For this review, take the finished solid that the model builds, in its own axes (mm). Face numbers are marked on the shaded views. A direction names the side the tool comes from. Round coordinates to 2 decimals unless told otherwise and drop trailing zeros. Loops run counter-clockwise (first coordinate to the right, second up) from the corner with the lowest first, then second, coordinate; pieces in that order, holes last. Notation, with made-up numbers: (-38.5, 53.25) -> (-26.5, 53.25) arc R28 cw to (-26.5, 91.25) -> close; hole circle Ø3 at (16.25, -18). An arc over 180 degrees is marked (long way). One line per question, with ' | ' between items. Start each with the question number.
1. Consider section A-A (x = -139.7). Write out the cut boundary in (y, z) (3 decimals).
2. Consider section B-B (z = -25.4). Write out the cut boundary in (x, y) (3 decimals), and give its area (3 significant figures).
3. Consider section C-C (x = -158.75). Write out the cut boundary in (y, z) (3 decimals).
4. For the marked faces 1 and 2, list the 3-axis set-ups (+Z, -Z, +X, -X, +Y, -Y) from which the entire face can be reached by the end or side of a thin tool; tool diameter is ignored.
5. Consider section D-D (z = -33.5). Write out the cut boundary in (x, y) (3 decimals), and give its area (3 significant figures).
6. For pin 1 Ø22 at (x, y) = (-52, 19.5) entering from +Z (3 decimals); pin 2 Ø2 at (x, z) = (-70.5, -23.5) entering from +Y, all flat-tipped, find the tip position at first contact; note any pin that passes through.
7. Wall thickness on line 1 along Z through (x, y) = (-149, 38) (3 decimals); line 2 along Y through (x, z) = (-156, -11.5) (3 decimals); line 3 along Z through (x, y) = (-64, 0.5): over which ranges is each line inside the solid? List them lowest first.
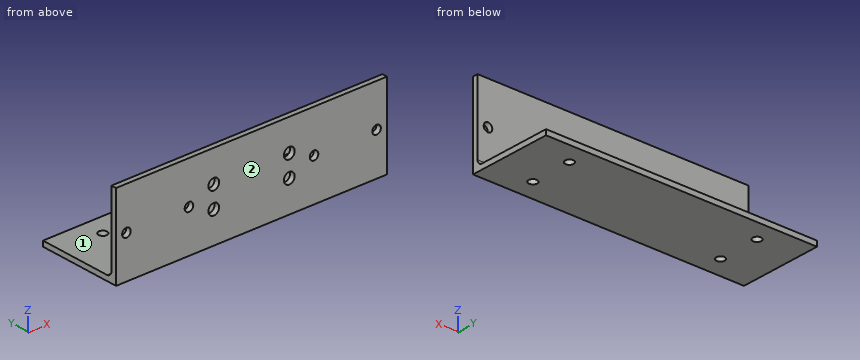
```python
from build123d import *

# Parameters (mm, degrees)
F1_DEPTH = 165.1
F2_R     = 2.6162
F2_R_2   = 3.302
F3_DEPTH = 50.801
F4_R     = 2.6162
F5_DEPTH = 25.4


with BuildPart() as f1:
    # F0 (on Right) → F1 (new body)
    with BuildSketch(Plane.YZ):
        with BuildLine():
            Line((0, -44.45), (0, 0))
            Line((0, 0), (-3.175, 0))
            Line((-3.175, 0), (-3.175, -50.8))
            Line((-3.175, -50.8), (47.625, -50.8))
            Line((47.625, -50.8), (47.625, -47.625))
            Line((47.625, -47.625), (3.175, -47.625))
            ThreePointArc((3.175, -47.625), (0.929936, -46.695064), (0, -44.45))
        make_face()
    extrude(amount=-F1_DEPTH)

    # F2 (on face) → F3 (cut, through all)
    with BuildSketch(Plane.XZ.offset(3.175)):
        with Locations((-158.75, -25.4)):
            Circle(F2_R)
        with Locations((-120.65, -25.4)):
            Circle(F2_R)
        with Locations((-44.45, -25.4)):
            Circle(F2_R)
        with Locations((-6.35, -25.4)):
            Circle(F2_R)
        with Locations((-59.5503, -31.9024)):
            Circle(F2_R_2)
        with Locations((-105.5497, -31.9024)):
            Circle(F2_R_2)
        with Locations((-59.5503, -18.8976)):
            Circle(F2_R_2)
        with Locations((-105.5497, -18.8976)):
            Circle(F2_R_2)
    extrude(amount=-F3_DEPTH, mode=Mode.SUBTRACT)

    # F4 (on face) → F5 (cut)
    with BuildSketch(Plane(origin=(0, 0, -50.8), x_dir=(1, 0, 0), z_dir=(0, 0, -1))):
        with Locations((-25.4, -34.925)):
            Circle(F4_R)
        with Locations((-25.4, -9.525)):
            Circle(F4_R)
        with Locations((-139.7, -34.925)):
            Circle(F4_R)
        with Locations((-139.7, -9.525)):
            Circle(F4_R)
    extrude(amount=-F5_DEPTH, mode=Mode.SUBTRACT)


solid = f1.part
```
Answer block:
1) outline: (-3.175, -50.8) -> (6.909, -50.8) -> (6.909, -47.625) -> (3.175, -47.625) arc R3.175 cw to (0, -44.45) -> (0, 0) -> (-3.175, 0) -> close; (12.141, -50.8) -> (32.309, -50.8) -> (32.309, -47.625) -> (12.141, -47.625) -> close; (37.541, -50.8) -> (47.625, -50.8) -> (47.625, -47.625) -> (37.541, -47.625) -> close
2) outline: (-165.1, -3.175) -> (-161.366, -3.175) -> (-161.366, 0) -> (-165.1, 0) -> close; (-156.134, -3.175) -> (-123.266, -3.175) -> (-123.266, 0) -> (-156.134, 0) -> close; (-118.034, -3.175) -> (-47.066, -3.175) -> (-47.066, 0) -> (-118.034, 0) -> close; (-41.834, -3.175) -> (-8.966, -3.175) -> (-8.966, 0) -> (-41.834, 0) -> close; (-3.734, -3.175) -> (0, -3.175) -> (0, 0) -> (-3.734, 0) -> close | area: 458 mm2
3) outline: (-3.175, -50.8) -> (47.625, -50.8) -> (47.625, -47.625) -> (3.175, -47.625) arc R3.175 cw to (0, -44.45) -> (0, -28.016) -> (-3.175, -28.016) -> close; (-3.175, -22.784) -> (0, -22.784) -> (0, 0) -> (-3.175, 0) -> close
4) face 1: +Z, +X, -X, +Y | face 2: +Z, -Z, +X, -X, -Y
5) outline: (-165.1, -3.175) -> (-108.439, -3.175) -> (-108.439, 0) -> (-165.1, 0) -> close; (-102.66, -3.175) -> (-62.44, -3.175) -> (-62.44, 0) -> (-102.66, 0) -> close; (-56.661, -3.175) -> (0, -3.175) -> (0, 0) -> (-56.661, 0) -> close | area: 487 mm2
6) pin 1: stops at z = -47.625 | pin 2: stops at y = 0
7) line 1: z = -50.8 to -47.625 | line 2: y = -3.175 to 0 | line 3: z = -50.8 to -46.16
